Work out the finished part from the listing and answer in its coordinate system (mm). A direction names the side the tool comes from. Coordinates: 2 decimals unless noted, no trailing zeros. Loops run counter-clockwise (first coordinate to the right, second up) from the corner with the lowest first, then second, coordinate; pieces in that order, holes last. Notation, with made-up numbers: (78, 12.5) - (130, 12.5) arc R32 ccw to (130, 41.5) - close; hole circle Ø8 at (-23, -32.75). An arc over 180 degrees is marked (long way). Write each question's results on one line, items separated by ' | '. Start each with the question number.
Item 1: Consider probe 1 along Z at (x, y) = (180, 9); probe 2 along X at (y, z) = (5, 0); probe 3 along X at (y, z) = (15.9, 0). Determine where each line is inside the solid, lowest interval first. Write a range as [from, to].
Item 2: A tool of negligible diameter and unlimited length cuts with its end or side. For faces 5 (the face through (-5, 18, 0)), 6 (the face through (172.19, 16.03, -1.73)), from which of +Z, -Z, +X, -X, +Y, -Y can it reach the whole face along a straight path? Write none if from no direction.
Item 3: For a pull along X with two mould halves and no side action, classify faces 1 (the face through (184, 14, 2)), 2 (the face through (183.966, 6.902, -0.521)), 3 (the face through (195, 9, 0)), 4 (the face through (-13, 9, 15)) as +X half, -X half, draft (parallel to the pull), parting line (faces both ways), or undercut.
Item 4: Section A-A, the plane z = 0 is taken. Write down the section's boundary in (x, y), plus the area to 3 significant figures.
from build123d import *

# Parameters (mm, degrees)
SKETCH1_R           = 4
BOSS_EXTRUDE1_DEPTH = 18
SKETCH2_R           = 8
CUT_EXTRUDE1_DEPTH  = 4


with BuildPart() as part:
    # Sketch1 → Boss-Extrude1 (new body)
    with BuildSketch(Plane(origin=(0, 0, 0), x_dir=(1, 0, 0), z_dir=(0, 1, 0))):
        with BuildLine():
            Line((-200, 15), (-200, -15))
            Line((-200, -15), (180, -15))
            ThreePointArc((180, -15), (195, 0), (180, 15))
            Line((180, 15), (-200, 15))
        make_face()
        with Locations(Location((180, 0, 0), (0, 0, 270))):
            Circle(SKETCH1_R, mode=Mode.SUBTRACT)
    extrude(amount=BOSS_EXTRUDE1_DEPTH)

    # Sketch2 → Cut-Extrude1 (cut)
    with BuildSketch(Plane(origin=(0, 18, 0), x_dir=(1, 0, 0), z_dir=(0, 1, 0))):
        with Locations(Location((180, 0, 0), (0, 0, 270))):
            Circle(SKETCH2_R)
    extrude(amount=-CUT_EXTRUDE1_DEPTH, mode=Mode.SUBTRACT)


solid = part.part
Answer key:
1) probe 1: z = [-15, -4], [4, 15] | probe 2: x = [-200, 176], [184, 195] | probe 3: x = [-200, 172], [188, 195]
2) face 5: +Z, -Z, +X, -X, +Y | face 6: +Y
3) face 1: undercut | face 2: undercut | face 3: +X half | face 4: draft
4) outline: (-200, 0) - (176, 0) - (176, 14) - (172, 14) - (172, 18) - (-200, 18) - close; (184, 0) - (195, 0) - (195, 18) - (188, 18) - (188, 14) - (184, 14) - close | area: 6,930 mm^2
